```python
from build123d import *

# Parameters (mm, degrees)
SKETCH2_R          = 0.5
CUT_EXTRUDE1_DEPTH = 18


with BuildPart() as part:
    # Sketch1 → Revolve1 (revolve)
    with BuildSketch(Plane.XY):
        Polygon((0, 0), (10, 0), (37.25, 9.918188884), (37.25, 13.110722201), (36.22393957, 12.737266746), (9.471019058, 3), (0, 3), align=None)
    revolve(axis=Axis((0, 0, 0), (0, 1, 0)))

    # Sketch2 → Cut-Extrude1 (cut)
    with BuildSketch(Plane(origin=(0, 3, 0), x_dir=(1, 0, 0), z_dir=(0, 1, 0))):
        with Locations((0, 4.735509529)):
            Circle(SKETCH2_R)
        Circle(SKETCH2_R)
        with Locations((4.503737195, 1.463352921)):
            Circle(SKETCH2_R)
        with Locations((2.783462663, -3.831107686)):
            Circle(SKETCH2_R)
        with Locations((-2.783462663, -3.831107686)):
            Circle(SKETCH2_R)
        with Locations((-4.503737195, 1.463352921)):
            Circle(SKETCH2_R)
    extrude(amount=-CUT_EXTRUDE1_DEPTH, mode=Mode.SUBTRACT)


solid = part.part
```
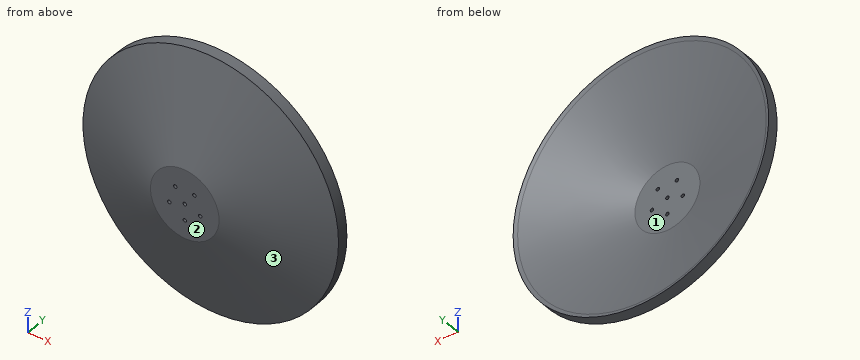
Work out the finished part from the listing and answer in its coordinate system (mm). Face numbers are marked on the shaded views. Coordinates: 2 decimals unless noted, no trailing zeros. Answer as a JSON object with one key per item and string values.
1. The mould has two halves that part along X. Classify the marked faces 1, 2 and 3: +X half, -X half, draft (parallel to the pull), parting line (faces both ways), or undercut.
Output values:
{"face 1": "undercut", "face 2": "draft", "face 3": "parting line"}
2. Consider line 1 (Y direction, x = 0, z = -1.5); line 2 (Y direction, x = -5.5, z = -8.5). Determine where each line is inside the solid, lowest interval first.
Output values:
{"line 1": "y = 0 to 3", "line 2": "y = 0.05 to 3.24"}
3. Each of these flat-tipped pins is pushed along its axis until it touches: P1, Ø1, axis at x = -25, y = 11.5, coming from the -Z side; P2, Ø4, axis at x = 17, z = -24.5, coming from the -Y side; P3, Ø1.5, axis at x = -11.5, z = -25.5, coming from the -Y side. Where does it stop, or does it pass through?
Output values:
{"P1": "stops at z = -28.06", "P2": "stops at y = 6.49", "P3": "stops at y = 6.27"}
